```python
from build123d import *

# Parameters (mm, degrees)
BOSS_EXTRUDE1_DEPTH      = 27.5
BOSS_EXTRUDE2_START      = 3
BOSS_EXTRUDE2_DEPTH      = 3
SKETCH3_W                = 19
SKETCH3_H                = 6
BOSS_EXTRUDE3_DEPTH      = 4
M3_CLEARANCE_HOLE1_D     = 3.2
M3_CLEARANCE_HOLE1_DEPTH = 4
FILLET1_R                = 3
M3_CLEARANCE_HOLE2_D     = 3.6
FILLET2_R                = 2


with BuildPart() as part:
    # Sketch1 → Boss-Extrude1 (new body)
    with BuildSketch(Plane.XY):
        with BuildLine():
            Line((-3.5, 44), (-3.5, 39.846580782))
            ThreePointArc((-3.5, 39.846580782), (0, 40), (3.5, 39.846580782))
            Line((3.5, 39.846580782), (3.5, 44))
            Line((3.5, 44), (-3.5, 44))
        make_face()
    extrude(amount=BOSS_EXTRUDE1_DEPTH)

    # Sketch2 → Boss-Extrude2 (add)
    with BuildSketch(Plane(origin=(0, 0, 0), x_dir=(-1, 0, 0), z_dir=(0, 0, -1)).offset(BOSS_EXTRUDE2_START)):
        with BuildLine():
            ThreePointArc((-4.728025778, 35.688174123), (-5.364869156, 35.598008075), (-6, 35.496478699))
            Line((-6, 35.496478699), (-6, 33))
            Line((-6, 33), (6, 33))
            Line((6, 33), (6, 35.496478699))
            ThreePointArc((6, 35.496478699), (5.364869156, 35.598008075), (4.728025778, 35.688174123))
            ThreePointArc((4.728025778, 35.688174123), (2.998157551, 34.269097614), (1.540989958, 35.967003628))
            ThreePointArc((1.540989958, 35.967003628), (0, 36), (-1.540989958, 35.967003628))
            ThreePointArc((-1.540989958, 35.967003628), (-1.538452767, 35.915033888), (-1.537606739, 35.863009131))
            ThreePointArc((-1.537606739, 35.863009131), (-3.050058074, 34.265406167), (-4.728025778, 35.688174123))
        make_face()
        with BuildLine():
            Line((-3.5, 44), (-6, 44))
            Line((-6, 44), (-6, 35.496478699))
            ThreePointArc((-6, 35.496478699), (-5.364869156, 35.598008075), (-4.728025778, 35.688174123))
            ThreePointArc((-4.728025778, 35.688174123), (-3.277055927, 37.456920648), (-1.540989958, 35.967003628))
            ThreePointArc((-1.540989958, 35.967003628), (0, 36), (1.540989958, 35.967003628))
            ThreePointArc((1.540989958, 35.967003628), (3.189631496, 37.462163103), (4.737606739, 35.863009131))
            ThreePointArc((4.737606739, 35.863009131), (4.735209703, 35.775460466), (4.728025778, 35.688174123))
            ThreePointArc((4.728025778, 35.688174123), (5.364869156, 35.598008075), (6, 35.496478699))
            Line((6, 35.496478699), (6, 44))
            Line((6, 44), (3.5, 44))
            Line((3.5, 44), (3.5, 39.846580782))
            ThreePointArc((3.5, 39.846580782), (0, 40), (-3.5, 39.846580782))
            Line((-3.5, 39.846580782), (-3.5, 44))
        make_face()
        with BuildLine():
            Line((-3.5, 44), (-3.5, 39.846580782))
            ThreePointArc((-3.5, 39.846580782), (0, 40), (3.5, 39.846580782))
            Line((3.5, 39.846580782), (3.5, 44))
            Line((3.5, 44), (-3.5, 44))
        make_face()
    extrude(amount=-BOSS_EXTRUDE2_DEPTH)

    # Sketch3 → Boss-Extrude3 (add)
    with BuildSketch(Plane.XY.offset(27.5)):
        with Locations((0, 41)):
            Rectangle(SKETCH3_W, SKETCH3_H)
    extrude(amount=-BOSS_EXTRUDE3_DEPTH)

    # M3 Clearance Hole1
    with Locations(Plane.XY.offset(27.5)):
        with Locations((-6.25, 41), (6.25, 41)):
            Hole(M3_CLEARANCE_HOLE1_D / 2, depth=M3_CLEARANCE_HOLE1_DEPTH)

    # Fillet1
    fillet1_edges = [part.edges().sort_by_distance(p)[0] for p in [
        (9.5, 38, 25.5),
        (9.5, 44, 25.5),
        (-9.5, 38, 25.5),
        (-9.5, 44, 25.5),
    ]]
    fillet(fillet1_edges, radius=FILLET1_R - 0.0001)  # a hair under: the kernel refuses the full size

    # M3 Clearance Hole2 (through all)
    with Locations(Plane(origin=(0, 44, 0), x_dir=(1, 0, 0), z_dir=(0, 1, 0))):
        with Locations((0, -15)):
            Hole(M3_CLEARANCE_HOLE2_D / 2)

    # Fillet2
    fillet2_edges = [part.edges().sort_by_distance(p)[0] for p in [
        (-6, 44, -1.5),
        (6, 44, -1.5),
    ]]
    fillet(fillet2_edges, radius=FILLET2_R)


solid = part.part
```
Input: part model. Units: mm. Frame: model coordinates. A direction names the side the tool comes from. Coordinates: 2 decimals unless noted, no trailing zeros. Order: outer loops, then holes, each group sorted by start corner. A loop starts at its lowest first (then second) coordinate and runs counter-clockwise, first axis right, second up. Notation, with made-up numbers: (15, 81.25) - (33, 81.25) arc R24 ccw to (33, 106.25) - close; hole circle Ø10 at (-37.75, 45). An arc over 180 degrees is marked (long way). Return JSON: item names as keys, results as strings.
Q1. Cut plane A-A (y = 41.5). Return loops of the section in (x, z), then the cut area to 3 significant figures.
The answers:
{"outline": "(-9.46, 23.5) - (-7.77, 23.5) - (-7.77, 27.5) - (-9.46, 27.5) - close; (-6, -3) - (6, -3) - (6, 0) - (3.5, 0) - (3.5, 23.5) - (4.73, 23.5) - (4.73, 27.5) - (-4.73, 27.5) - (-4.73, 23.5) - (-3.5, 23.5) - (-3.5, 0) - (-6, 0) - close; (7.77, 23.5) - (9.46, 23.5) - (9.46, 27.5) - (7.77, 27.5) - close; hole circle Ø3.6 at (0, 15)", "area": "242 mm2"}
Q2. First-contact query: pin 1 (5 mm diameter, centred on x = 6.25, y = 41, fed in from +Z); pin 2 (2.5 mm diameter, centred on y = 36, z = -1.5, fed in from +X); pin 3 (4.5 mm diameter, centred on x = -1.5, z = 26.5, fed in from -Y); pin 4 (4.5 mm diameter, centred on y = 41.5, z = 8, fed in from +X). Flat tips, straight axial feed; report the tip coordinate or a pass-through.
The answers:
{"pin 1": "stops at z = 27.5", "pin 2": "stops at x = 6", "pin 3": "stops at y = 38", "pin 4": "stops at x = 3.5"}
Q3. Access query for faces 4 (the cylindrical face through (-6.99, 39.58, 25.47)), 5 (the flat face through (3.5, 42, 12)), 6 (the cylindrical face through (-5.4, 43.43, -1.48)), 7 (the cylindrical face through (5.4, 43.43, -1.48)), 8 (the flat face through (0, 38, 26)). Directions: +Z, -Z, +X, -X, +Y, -Y. A direction counts if a zero-diameter tool reaches every point of the face in a straight line with its end or side. Return the directions, or none.
The answers:
{"face 4": "+Z", "face 5": "+X, +Y, -Y", "face 6": "-Z, -X, +Y", "face 7": "-Z, +X, +Y", "face 8": "+Z, +X, -X, -Y"}
Q4. Draft query along Z for faces 1 (the cylindrical face through (0, 40, 12)), 2 (the flat face through (0, 39, -3)), 3 (the cylindrical face through (8.6, 43.14, 25.47)). Return one class per face: +Z half, -Z half, draft (parallel to the pull), parting line (faces both ways), or undercut.
The answers:
{"face 1": "undercut", "face 2": "-Z half", "face 3": "draft"}
Q5. Cut plane C-C (x = 0). Return loops of the section in (y, z), then the cut area to 3 significant figures.
The answers:
{"outline": "(33, -3) - (44, -3) - (44, 13.2) - (40, 13.2) - (40, 0) - (33, 0) - close; (38, 23.5) - (40, 23.5) - (40, 16.8) - (44, 16.8) - (44, 27.5) - (38, 27.5) - close", "area": "137 mm2"}
Q6. Cut plane D-D (z = 25). State how many separate pieces and enclosed holes the cut face has, then the cut area to 3 significant figures.
The answers:
{"separate pieces": "1", "enclosed holes": "2", "area": "90.2 mm2"}
Q7. Ray query, probe 1 along Z at (x, y) = (-4, 43.75); probe 2 along X at (y, z) = (36, -1.5); probe 3 along X at (y, z) = (40.85, 15). Return the intervals inside material, ascending.
The answers:
{"probe 1": "z = -3 to 0, 23.5 to 27.5", "probe 2": "x = -6 to -4.73, -1.54 to 1.54, 4.73 to 6", "probe 3": "x = -3.5 to -1.8, 1.8 to 3.5"}
Q8. Cut plane B-B (z = 15). Return loops of the section in (x, y), then the cut area to 3 significant figures.
The answers:
{"outline": "(-3.5, 39.85) arc R40 cw to (-1.8, 39.96) - (-1.8, 44) - (-3.5, 44) - close; (1.8, 39.96) arc R40 cw to (3.5, 39.85) - (3.5, 44) - (1.8, 44) - close", "area": "13.9 mm2"}
